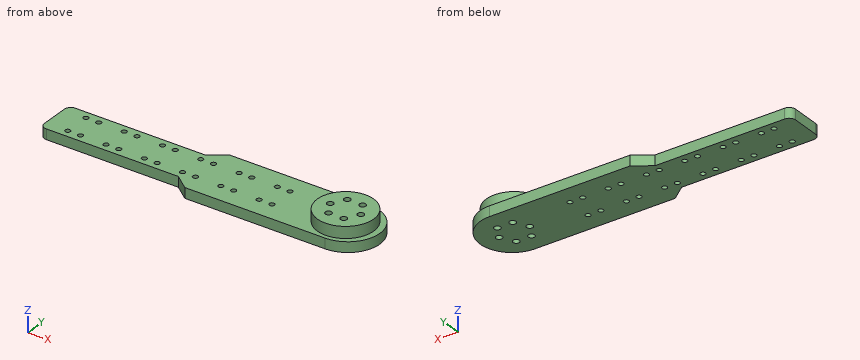
from build123d import *

# Parameters (mm, degrees)
SKETCH_1_R          = 2
EXTRUDE_1_DEPTH     = 8
FILLET_1_R          = 10
SKETCH_2_R          = 22
SKETCH_2_R_2        = 2.5
EXTRUDE_3_DEPTH     = 9
MM_1_D              = 5
SKETCH_11_W         = 120
SKETCH_11_H         = 9.00000035
CUT_EXTRUDE_2_DEPTH = 143.499121284
FILLET_5_R          = 5
FILLET_8_R          = 5
RIB_9_REACH         = 145.227
SKETCH_14_WALL_W    = 304.68091252
SKETCH_14_WALL_H    = 8
RIB_26_REACH        = 144.499
SKETCH_16_WALL_W    = 14.607309972
SKETCH_16_WALL_H    = 8


with BuildPart() as part:
    # 草图1 → 凸台-拉伸1 (new body)
    with BuildSketch(Plane.XY):
        with BuildLine():
            Line((-114.99999839, -24.99999965), (114.99999517, -24.99999965))
            ThreePointArc((114.99999517, -24.99999965), (139.99999839, -2.87e-06), (115.00000161, 25.00000035))
            Line((115.00000161, 25.00000035), (-114.99999839, 25.00000035))
            Line((-114.99999839, 25.00000035), (-114.99999839, -24.99999965))
        make_face()
        with Locations((-67.422337314, 10.00000035)):
            Circle(SKETCH_1_R, mode=Mode.SUBTRACT)
        with Locations(Location((-67.422337314, -9.99999965, 0), (0, 0, 180))):
            Circle(SKETCH_1_R, mode=Mode.SUBTRACT)
        with Locations((-57.422337314, 10.00000035)):
            Circle(SKETCH_1_R, mode=Mode.SUBTRACT)
        with Locations(Location((-57.422337314, -9.99999965, 0), (0, 0, 180))):
            Circle(SKETCH_1_R, mode=Mode.SUBTRACT)
        with Locations((-37.422337314, 10.00000035)):
            Circle(SKETCH_1_R, mode=Mode.SUBTRACT)
        with Locations((-27.422337314, 10.00000035)):
            Circle(SKETCH_1_R, mode=Mode.SUBTRACT)
        with Locations(Location((-37.422337314, -9.99999965, 0), (0, 0, 180))):
            Circle(SKETCH_1_R, mode=Mode.SUBTRACT)
        with Locations(Location((-27.422337314, -9.99999965, 0), (0, 0, 180))):
            Circle(SKETCH_1_R, mode=Mode.SUBTRACT)
        with Locations((-7.422337314, 10.00000035)):
            Circle(SKETCH_1_R, mode=Mode.SUBTRACT)
        with Locations((2.577662686, 10.00000035)):
            Circle(SKETCH_1_R, mode=Mode.SUBTRACT)
        with Locations(Location((-7.422337314, -9.99999965, 0), (0, 0, 180))):
            Circle(SKETCH_1_R, mode=Mode.SUBTRACT)
        with Locations(Location((2.577662686, -9.99999965, 0), (0, 0, 180))):
            Circle(SKETCH_1_R, mode=Mode.SUBTRACT)
        with Locations((22.577662686, 10.00000035)):
            Circle(SKETCH_1_R, mode=Mode.SUBTRACT)
        with Locations((32.577662686, 10.00000035)):
            Circle(SKETCH_1_R, mode=Mode.SUBTRACT)
        with Locations(Location((22.577662686, -9.99999965, 0), (0, 0, 180))):
            Circle(SKETCH_1_R, mode=Mode.SUBTRACT)
        with Locations(Location((32.577662686, -9.99999965, 0), (0, 0, 180))):
            Circle(SKETCH_1_R, mode=Mode.SUBTRACT)
        with Locations((-97.422337314, 10.00000035)):
            Circle(SKETCH_1_R, mode=Mode.SUBTRACT)
        with Locations(Location((-97.422337314, -9.99999965, 0), (0, 0, 180))):
            Circle(SKETCH_1_R, mode=Mode.SUBTRACT)
        with Locations((-87.422337314, 10.00000035)):
            Circle(SKETCH_1_R, mode=Mode.SUBTRACT)
        with Locations(Location((-87.422337314, -9.99999965, 0), (0, 0, 180))):
            Circle(SKETCH_1_R, mode=Mode.SUBTRACT)
        with Locations((52.577662686, 10.00000035)):
            Circle(SKETCH_1_R, mode=Mode.SUBTRACT)
        with Locations((62.577662686, 10.00000035)):
            Circle(SKETCH_1_R, mode=Mode.SUBTRACT)
        with Locations(Location((52.577662686, -9.99999965, 0), (0, 0, 180))):
            Circle(SKETCH_1_R, mode=Mode.SUBTRACT)
        with Locations(Location((62.577662686, -9.99999965, 0), (0, 0, 180))):
            Circle(SKETCH_1_R, mode=Mode.SUBTRACT)
    extrude(amount=EXTRUDE_1_DEPTH)

    # 圆角1
    fillet_1_edges = [part.edges().sort_by_distance(p)[0] for p in [
        (-114.99999839, -24.99999965, 4),
        (-114.99999839, 25.00000035, 4),
    ]]
    fillet(fillet_1_edges, radius=FILLET_1_R)

    # 草图2 → 凸台-拉伸3 (add)
    with BuildSketch(Plane.XY.offset(8)):
        with Locations(Location((113.184869064, 3.5e-07, 0), (0, 0, 180))):
            Circle(SKETCH_2_R)
        with Locations((119.184869064, -10.392304495)):
            Circle(SKETCH_2_R_2, mode=Mode.SUBTRACT)
        with Locations((107.184869064, -10.392304495)):
            Circle(SKETCH_2_R_2, mode=Mode.SUBTRACT)
        with Locations((101.184869064, 3.5e-07)):
            Circle(SKETCH_2_R_2, mode=Mode.SUBTRACT)
        with Locations((107.184869064, 10.392305195)):
            Circle(SKETCH_2_R_2, mode=Mode.SUBTRACT)
        with Locations((119.184869064, 10.392305195)):
            Circle(SKETCH_2_R_2, mode=Mode.SUBTRACT)
        with Locations((125.184869064, 3.5e-07)):
            Circle(SKETCH_2_R_2, mode=Mode.SUBTRACT)
    extrude(amount=EXTRUDE_3_DEPTH)

    # 大小mm 暗销孔1 (through all)
    with Locations(Plane.XY.offset(8)):
        with Locations((119.184869064, -10.392304495), (107.184869064, -10.392304495), (101.184869064, 3.5e-07), (107.184869064, 10.392305195), (119.184869064, 10.392305195), (125.184869064, 3.5e-07)):
            Hole(MM_1_D / 2)

    # 草图11 → 切除-拉伸2 (cut, through all)
    with BuildSketch(Plane.XY.offset(8)):
        with Locations((-54.99999839, 20.500000175)):
            Rectangle(SKETCH_11_W, SKETCH_11_H)
        with Locations((-54.99999839, -20.500000175)):
            Rectangle(SKETCH_11_W, SKETCH_11_H)
    extrude(amount=-CUT_EXTRUDE_2_DEPTH, mode=Mode.SUBTRACT)

    # 圆角5
    fillet_5_edges = [part.edges().sort_by_distance(p)[0] for p in [
        (-114.949872796, 16, 4),
    ]]
    fillet(fillet_5_edges, radius=FILLET_5_R)

    # 圆角8
    fillet_8_edges = [part.edges().sort_by_distance(p)[0] for p in [
        (-114.949872726, -16, 4),
    ]]
    fillet(fillet_8_edges, radius=FILLET_8_R)

    # 草图14 wall → 筋9 (add, up to next)
    with BuildSketch(Plane(origin=(-1.751049722, 20.500000175, 0), x_dir=(-0.832090153066, -0.554640403479, 0), z_dir=(-0.554640403479, 0.832090153066, 0)), mode=Mode.PRIVATE) as rib_9_sk1:
        with Locations((0, 4)):
            Rectangle(SKETCH_14_WALL_W, SKETCH_14_WALL_H)
    rib_9_tool1 = extrude(rib_9_sk1.sketch, amount=-RIB_9_REACH, mode=Mode.PRIVATE) - part.part
    add(rib_9_tool1.solids().sort_by_distance((-1.751049722, 20.500000175, 0))[0])

    # 草图16 wall → 筋26 (add, up to next)
    with BuildSketch(Plane(origin=(-0.75268251, -20.500000175, 8), x_dir=(-0.787644560259, 0.616129894336, 0), z_dir=(-0.616129894336, -0.787644560259, 0)), mode=Mode.PRIVATE) as rib_26_sk1:
        with Locations((0, 4)):
            Rectangle(SKETCH_16_WALL_W, SKETCH_16_WALL_H)
    rib_26_tool1 = extrude(rib_26_sk1.sketch, amount=-RIB_26_REACH, mode=Mode.PRIVATE) - part.part
    add(rib_26_tool1.solids().sort_by_distance((-0.75268251, -20.500000175, 8))[0])


solid = part.part
Work out the finished part from the listing and answer in its coordinate system (mm). Round coordinates to 2 decimals unless told otherwise and drop trailing zeros. Write each loop counter-clockwise with the first axis right and the second up, starting at its lowest first coordinate (ties: lowest second). Pieces come first, ordered by that corner, then holes. Notation, with made-up numbers: (18, -20.5) -> (22, -20.5) arc R13 ccw to (22, -10.5) -> close; hole circle Ø3 at (-29.5, 56.25). An arc over 180 degrees is marked (long way). Answer as CSV lines item,"result". Start each with the question number.
(1) The part is cut by section C-C, the plane y = -19. Give the vertices of the cut face in (x, z), then the cut area to 3 significant figures.
(2) The part is cut by section D-D, the plane z = 4. Give the number of separate pieces and of enclosed holes in the cut face, then the cut area to 3 significant figures.
(3) The part is cut by section B-B, the plane x = 68. Give the vertices of the cut face in (y, z).
(4) Each of these flat-tipped pins is pushed along its axis until it touches: pin 1 (2.5 mm diameter, centred on x = -67.42, y = 10, fed in from +Z); pin 2 (6 mm diameter, centred on x = 8, y = -0.5, fed in from +Z); pin 3 (4 mm diameter, centred on x = -39, z = 5.5, fed in from +Y); pin 4 (6 mm diameter, centred on y = 12.5, z = 7, fed in from +X). Where does it stop, or does it pass through?
(5) The part is cut by section A-A, the plane z = 14.25. Give the vertices of the cut face in (x, y), then the cut area to 3 significant figures.
(6) Find the intervals of material crossed by probe 1 along Y at (x, z) = (120, 6.25); probe 2 along X at (y, z) = (-12, 14.5); probe 3 along Y at (x, z) = (-23, 4), in increasing order.
Output values:
1,outline,"(-2.67, 0) -> (131.25, 0) -> (131.25, 8) -> (124.28, 8) -> (124.28, 17) -> (102.09, 17) -> (102.09, 8) -> (-2.67, 8) -> close"
1,area,"1,270 mm²"
2,separate pieces,"1"
2,enclosed holes,"30"
2,area,"10,000 mm²"
3,outline,"(-25, 0) -> (25, 0) -> (25, 8) -> (-25, 8) -> close"
4,pin 1,"passes through"
4,pin 2,"stops at z = 8"
4,pin 3,"stops at y = 16"
4,pin 4,"stops at x = 138.12"
5,outline,"circle Ø44 at (113.18, 0); hole circle Ø5 at (101.18, 0); hole circle Ø5 at (107.18, -10.39); hole circle Ø5 at (107.18, 10.39); hole circle Ø5 at (119.18, -10.39); hole circle Ø5 at (119.18, 10.39); hole circle Ø5 at (125.18, 0)"
5,area,"1,400 mm²"
6,probe 1,"y = -24.49 to -12.76, -8.03 to 8.03, 12.76 to 24.49"
6,probe 2,"x = 94.75 to 105.27, 109.1 to 117.27, 121.1 to 131.62"
6,probe 3,"y = -16 to 16"
